from build123d import *

# Parameters (mm, degrees)
F0_W      = 76.2
F0_H      = 25.4
F1_DEPTH  = 1.016
F1_FACE_W = 76.2
F1_FACE_H = 25.4
F2_DEPTH  = 15.24
F3_W      = 12.7
F3_H      = 12.7
F4_DEPTH  = 10.16


with BuildPart() as f1:
    # F0 (on Top) → F1 (new body)
    with BuildSketch(Plane.XY):
        with Locations((-38.1, 12.7)):
            Rectangle(F0_W, F0_H)
    extrude(amount=F1_DEPTH)

    # F1_face (on face) → F2 (join)
    with BuildSketch(Plane(origin=(-38.1, 12.7, 1.016), x_dir=(1, 0, 0), z_dir=(0, 0, 1))):
        Rectangle(F1_FACE_W, F1_FACE_H)
    extrude(amount=F2_DEPTH)

    # F3 (on face) → F4 (cut)
    with BuildSketch(Plane.XY.offset(16.256)):
        with Locations((-41.178353, 10.822336)):
            Rectangle(F3_W, F3_H)
    extrude(amount=-F4_DEPTH, mode=Mode.SUBTRACT)


solid = f1.part
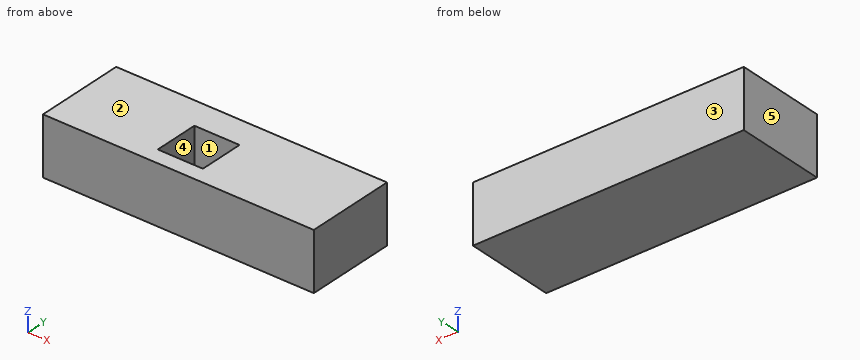
Could you check a few things on this model? Use its own coordinates, in mm. Face numbers are marked on the shaded views. A direction names the side the tool comes from. Round coordinates to 2 decimals unless told otherwise and drop trailing zeros. Write each loop counter-clockwise with the first axis right and the second up, starting at its lowest first coordinate (ties: lowest second). Pieces come first, ordered by that corner, then holes. Notation, with made-up numbers: (84, 42.5) -> (93, 42.5) arc R25 cw to (93, 78.5) -> close; hole circle Ø5 at (-40, 63). An arc over 180 degrees is marked (long way). Use a Markdown table: item, result.
1. If we section it at C-C (y = 14.25): List the corners of the cut face in (x, z) for me.
Answer key:
| item | result |
|---|---|
| outline | (-76.2, 0) -> (0, 0) -> (0, 16.26) -> (-34.83, 16.26) -> (-34.83, 6.1) -> (-47.53, 6.1) -> (-47.53, 16.26) -> (-76.2, 16.26) -> close |
2. Which directions (+Z, -Z, +X, -X, +Y, -Y) give clear straight access to the entire face, cutting with the end or side of a thin tool? Please do the marked faces 1 and 2.
Answer key:
| item | result |
|---|---|
| face 1 | +Z |
| face 2 | +Z, +X, -X, +Y, -Y |
3. If we section it at A-A (z = 9): List the corners of the cut face in (x, y) for me, then the cut area to 3 significant figures.
Answer key:
| item | result |
|---|---|
| outline | (-76.2, 0) -> (0, 0) -> (0, 25.4) -> (-76.2, 25.4) -> close; hole (-47.53, 4.47) -> (-34.83, 4.47) -> (-34.83, 17.17) -> (-47.53, 17.17) -> close |
| area | 1,770 mm^2 |
4. If we section it at B-B (x = -41): List the corners of the cut face in (y, z) for me.
Answer key:
| item | result |
|---|---|
| outline | (0, 0) -> (25.4, 0) -> (25.4, 16.26) -> (17.17, 16.26) -> (17.17, 6.1) -> (4.47, 6.1) -> (4.47, 16.26) -> (0, 16.26) -> close |
5. We'd pull the mould along X, two halves only. Please class the marked faces 3, 4 and 5: +X half, -X half, draft (parallel to the pull), parting line (faces both ways), or undercut.
Answer key:
| item | result |
|---|---|
| face 3 | draft |
| face 4 | undercut |
| face 5 | -X half |
6. Please list where these lines run through material, in increasing order: probe 1 along X at (y, z) = (7.25, 14.5); probe 2 along Y at (x, z) = (-37.5, 9).
Answer key:
| item | result |
|---|---|
| probe 1 | x = -76.2 to -47.53, -34.83 to 0 |
| probe 2 | y = 0 to 4.47, 17.17 to 25.4 |
